from build123d import *

# Parameters (mm, degrees)
SKETCH1_R               = 20
BOSS_EXTRUDE1_DEPTH     = 40
CUT_EXTRUDE1_DEPTH      = 15
SKETCH3_R               = 2
CUT_EXTRUDE2_DEPTH      = 15
CUT_EXTRUDE3_DEPTH      = 9
SKETCH5_R               = 2.5
CUT_EXTRUDE4_DEPTH      = 23.925000127
CUT_EXTRUDE4_DEPTH_BACK = 18.0750001
SKETCH6_W               = 10.42
SKETCH6_H               = 6.18
CUT_EXTRUDE5_DEPTH      = 15
SKETCH7_R               = 2
CUT_EXTRUDE6_DEPTH      = 15
CUT_EXTRUDE6_DEPTH_BACK = 10


with BuildPart() as part:
    # Sketch1 → Boss-Extrude1 (new body)
    with BuildSketch(Plane(origin=(0, 0, 0), x_dir=(1, 0, 0), z_dir=(0, 1, 0))):
        Circle(SKETCH1_R)
    extrude(amount=BOSS_EXTRUDE1_DEPTH)

    # Sketch2 → Cut-Extrude1 (cut)
    with BuildSketch(Plane.XZ):
        with BuildLine():
            Line((-4.000002932, 5), (3.999997068, 5))
            add(Edge.make_bspline(
                [(3.999997068, 5), (8.199974497, 0.009249301), (3.999997068, -5)],
                knots=[0, 0, 0, 1, 1, 1], degree=2))
            Line((3.999997068, -5), (-4.000002932, -5))
            add(Edge.make_bspline(
                [(-4.000002932, 5), (-8.199982148, -0.00561634), (-4.000002932, -5)],
                knots=[0, 0, 0, 1, 1, 1], degree=2))
        make_face()
    extrude(amount=-CUT_EXTRUDE1_DEPTH, mode=Mode.SUBTRACT)

    # Sketch3 → Cut-Extrude2 (cut)
    with BuildSketch(Plane.XY.offset(-5)):
        with Locations((0, 12.004234523)):
            Circle(SKETCH3_R)
    extrude(amount=-CUT_EXTRUDE2_DEPTH, mode=Mode.SUBTRACT)

    # Sketch4 → Cut-Extrude3 (cut)
    with BuildSketch(Plane(origin=(0, 40, 0), x_dir=(1, 0, 0), z_dir=(0, 1, 0))):
        with BuildLine():
            Line((-3.75, 2.925), (3.75, 2.925))
            add(Edge.make_bspline(
                [(3.75, 2.925), (5.10000002, -3.7956e-05), (3.75, -2.925)],
                knots=[0, 0, 0, 1, 1, 1], degree=2))
            Line((3.75, -2.925), (-3.75, -2.925))
            add(Edge.make_bspline(
                [(-3.75, 2.925), (-5.10000002, -3.7956e-05), (-3.75, -2.925)],
                knots=[0, 0, 0, 1, 1, 1], degree=2))
        make_face()
    extrude(amount=-CUT_EXTRUDE3_DEPTH, mode=Mode.SUBTRACT)

    # Sketch5 → Cut-Extrude4 (cut, two sides)
    with BuildSketch(Plane(origin=(0, 0, 2.925), x_dir=(-1, 0, 0), z_dir=(0, 0, -1))) as cut_extrude4_sk:
        with Locations((0, 36)):
            Circle(SKETCH5_R)
    extrude(amount=CUT_EXTRUDE4_DEPTH, mode=Mode.SUBTRACT)
    extrude(cut_extrude4_sk.sketch, amount=-CUT_EXTRUDE4_DEPTH_BACK, mode=Mode.SUBTRACT)

    # Sketch6 → Cut-Extrude5 (cut)
    with BuildSketch(Plane.XZ):
        with Locations((0, 11.59)):
            Rectangle(SKETCH6_W, SKETCH6_H)
    extrude(amount=-CUT_EXTRUDE5_DEPTH, mode=Mode.SUBTRACT)

    # Sketch7 → Cut-Extrude6 (cut, two sides)
    with BuildSketch(Plane.XY.offset(8.5)) as cut_extrude6_sk:
        with Locations((0, 10.34)):
            Circle(SKETCH7_R)
    extrude(amount=CUT_EXTRUDE6_DEPTH, mode=Mode.SUBTRACT)
    extrude(cut_extrude6_sk.sketch, amount=-CUT_EXTRUDE6_DEPTH_BACK, mode=Mode.SUBTRACT)


solid = part.part
Verification items for the finished model (mm, model axes). A direction names the side the tool comes from. Coordinates: 2 decimals unless noted, no trailing zeros. Write each loop counter-clockwise with the first axis right and the second up, starting at its lowest first coordinate (ties: lowest second). Pieces come first, ordered by that corner, then holes. Notation, with made-up numbers: M -6.5,56 L 6.5,56 A13 ccw 6.5,72 Z; hole C 67,63.25 d9. An arc over 180 degrees is marked long. Use CSV: the item, a comma, the result in double quotes.
Q1. Thickness scan on line 1 along Y through (x, z) = (0, -14); line 2 along Y through (x, z) = (0, 17); line 3 along Z through (x, y) = (4, 10.5). Record the ranges inside material, lowest first. Write a range as [from, to].
Computed values:
line 1,"[0, 10], [14, 33.5], [38.5, 40]"
line 2,"[0, 8.34], [12.34, 33.5], [38.5, 40]"
line 3,"[-19.6, -5], [5, 8.5], [14.68, 19.6]"
Q2. Section check C-C, the plane z = 6. Enter the section's corners in (x, y), and give its area (3 significant figures).
Computed values:
outline,"M -19.08,0 L 19.08,0 L 19.08,40 L -19.08,40 Z; hole C 0,36 d5; hole C 0,10.34 d4"
area,"1,490 mm²"
Q3. Section check A-A, the plane x = 0. State how many separate pieces and enclosed holes the cut face has, and give its area (3 significant figures).
Computed values:
separate pieces,"6"
enclosed holes,"0"
area,"1,040 mm²"
Q4. Go/stop test with flat-tipped pins: P1, Ø3, axis at x = 0, y = 12, coming from the -Z side; P2, Ø1, axis at y = 22.5, z = -2, coming from the +X side; P3, Ø5, axis at y = 4.5, z = -5, coming from the +X side. Record where each tip stops, or that it passes through.
Computed values:
P1,"z = 5"
P2,"x = 19.94"
P3,"x = 19.84"
Q5. Section check B-B, the plane y = 25.5. Enter the section's corners in (x, z), and give its area (3 significant figures).
Computed values:
outline,"C 0,0 d40"
area,"1,260 mm²"
Q6. Mould release check, pull along Z, two halves, no side actions. Record for faces 4 (the cylindrical face through (-0.26, 12.323, 17.304)), 5 (the flat face through (-5.21, 7, 12)), 6 (the cylindrical face through (-4.336, 19.72, 19.524)): pulls with the +Z half, pulls with the -Z half, needs draft (parallel to the pull), parting line crosses it, or undercut.
Computed values:
face 4,"needs draft"
face 5,"undercut"
face 6,"parting line crosses it"
Q7. Set-up check for faces 1 (the flat face through (0, 7, 5)), 2 (the flat face through (0, 31, 0)), 3 (the cylindrical face through (-0.26, 12.323, 6.774)): record each of +Z, -Z, +X, -X, +Y, -Y from which the full face is reachable in a straight line by a thin tool's end or side.
Computed values:
face 1,"-Y"
face 2,"+Y"
face 3,"+Z"
